Answer from the drawing. Dimensions are ordinates in mm from the lowest x, y and z of the part. A direction names the side the tool comes from. Give positions to 0.01 mm unless a question says otherwise; leave off trailing zeros. Order: outer loops, then holes, each group sorted by start corner. A loop starts at its lowest first (then second) coordinate and runs counter-clockwise, first axis right, second up.
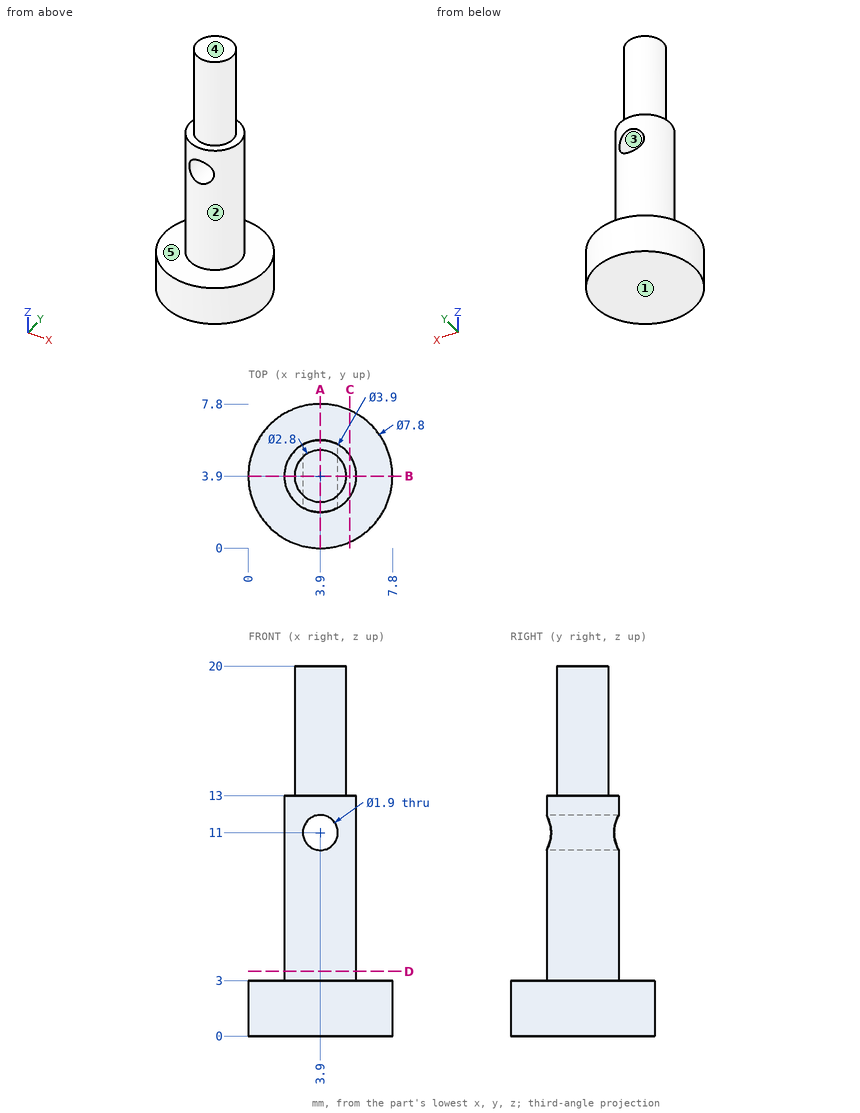
1) The part is cut by section B-B on y = 3.9. Determine the outline of the cut face in (x, z), and give its area (3 significant figures).
Final values:
outline: (0, 0) - (7.8, 0) - (7.8, 3) - (5.85, 3) - (5.85, 13) - (5.3, 13) - (5.3, 20) - (2.5, 20) - (2.5, 13) - (1.95, 13) - (1.95, 3) - (0, 3) - close; hole circle Ø1.9 at (3.9, 11)
area: 79.2 mm2
2) Given pin 1 (4 mm diameter, centred on y = 1.5, z = 8, fed in from +X); pin 2 (4 mm diameter, centred on y = 6, z = 17, fed in from +X); pin 3 (3 mm diameter, centred on x = 1, z = 12.5, fed in from +Y), each flat-ended and moving along its own axis, determine where each tip first touches the part or whether it passes through.
Final values:
pin 1: stops at x = 5.81
pin 2: stops at x = 5.3
pin 3: stops at y = 5.26
3) For a pull along X with two mould halves and no side action, classify the marked faces 1, 2 and 3 as released by +X, released by -X, zero draft, split by the parting line, or undercut.
Final values:
face 1: zero draft
face 2: split by the parting line
face 3: undercut
4) The part is cut by section A-A on x = 3.9. Determine the outline of the cut face in (y, z), and give its area (3 significant figures).
Final values:
outline: (0, 0) - (7.8, 0) - (7.8, 3) - (5.85, 3) - (5.85, 10.05) - (1.95, 10.05) - (1.95, 3) - (0, 3) - close; (1.95, 11.95) - (5.85, 11.95) - (5.85, 13) - (5.3, 13) - (5.3, 20) - (2.5, 20) - (2.5, 13) - (1.95, 13) - close
area: 74.6 mm2
5) A tool of negligible diameter and unlimited length cuts with its end or side. For the marked faces 4 and 5, from which of +Z, -Z, +X, -X, +Y, -Y can it reach the whole face along a straight path? Write none if from no direction.
Final values:
face 4: +Z, +X, -X, +Y, -Y
face 5: +Z
6) The part is cut by section D-D on z = 3.5. Determine the outline of the cut face in (x, y), and give its area (3 significant figures).
Final values:
outline: circle Ø3.9 at (3.9, 3.9)
area: 11.9 mm2
7) Consider L1, parallel to Z at x = 3.9, y = 3.9; L2, parallel to Z at x = 4.5, y = 0.5; L3, parallel to X at y = 3.2, z = 11. Determine where each line is inside the solid, lowest interval first.
Final values:
L1: z = 0 to 10.05, 11.95 to 20
L2: z = 0 to 3
L3: x = 2.08 to 2.95, 4.85 to 5.72
8) The part is cut by section C-C on x = 5.5. Determine the outline of the cut face in (y, z), and give its area (3 significant figures).
Final values:
outline: (0.34, 0) - (7.46, 0) - (7.46, 3) - (5.01, 3) - (5.01, 13) - (2.79, 13) - (2.79, 3) - (0.34, 3) - close
area: 43.6 mm2
